For this review, take the finished solid that the model builds, in its own axes (mm). A direction names the side the tool comes from. Give positions to 0.01 mm unless a question says otherwise; leave off trailing zeros. Write each loop counter-clockwise with the first axis right and the second up, starting at its lowest first coordinate (ties: lowest second). Pieces come first, ordered by that corner, then holes.
Q1. Insertion check: P1, Ø10, axis at x = -33, z = 9.5, coming from the -Y side; P2, Ø10, axis at y = 2.5, z = 15, coming from the -X side; P3, Ø1, axis at x = -34, z = 9.5, coming from the +Y side; P4, Ø11.5, axis at x = -44.45, y = 0, coming from the -Z side. Each pin has a flat end and moves straight along its axis. Give the tip position at first contact, or say it passes through.
Q2. We need section C-C (z = 8). Write out the cut boundary in (x, y), then the cut area to 3 significant figures.
Q3. We need section D-D (x = 4.5). Write out the cut boundary in (y, z).
Q4. Machinability: for faces 1 (the flat face through (35, -19.05, 6)), 2 (the flat face through (0, -14.288, 34)), 3 (the flat face through (-35, 19.05, 6)), 4 (the flat face through (-37, 0, 12.7)), which of the approach directions +Z, -Z, +X, -X, +Y, -Y give a long, thin tool a straight path to every point of the face, cutting with its end or side? Answer none if there is none.
Q5. For line 1 (Y direction, x = -44.45, z = 7.75); line 2 (Z direction, x = -50, y = 8.5); line 3 (Y direction, x = 50.5, z = 9), list the stretches that pass through material, from the lowest coordinate up.
Q6. We need section A-A (y = 0). Write out the cut boundary in (x, z).
Q7. Mouldability with a two-part tool opening along Y and no side actions: class faces 5 (the flat face through (35, 19.05, 6)), 6 (the flat face through (-35, -19.05, 6)), 7 (the flat face through (0, 0, 25.4)), 8 (the cylindrical face through (-37.636, 2.146, 6.439)) as released by +Y, released by -Y, zero draft, split by the parting line, or undercut.
Q8. We need section B-B (x = 50). Write out the cut boundary in (y, z).
```python
from build123d import *

# Parameters (mm, degrees)
F1_DEPTH = 31.75
F2_DEPTH = 19.05
F5_DEPTH = 12.7
F6_DEPTH = 25.4
F7_DEPTH = 25.4
F8_W     = 40.1893556118
F8_H     = 22.225
F8_W_2   = 32.2620980442
F9_DEPTH = 14.2875


with BuildPart() as f1:
    # F0 (on Front) → F1 (new body, symmetric)
    with BuildSketch(Plane.XZ):
        Polygon((0, 47.625), (0, 12.7), (20.1639581514, 12.7), align=None)
        Polygon((-27.4963065702, 0), (0, 0), (0, 12.7), (-20.1639581514, 12.7), align=None)
        Polygon((0, 12.7), (0, 0), (27.4963065702, 0), (20.1639581514, 12.7), align=None)
        Polygon((-20.1639581514, 12.7), (0, 12.7), (0, 47.625), align=None)
    extrude(amount=F1_DEPTH, both=True)

    # F0 (on Front) → F2 (join, symmetric)
    with BuildSketch(Plane.XZ):
        Polygon((-27.4963065702, 0), (0, 0), (0, 12.7), (-20.1639581514, 12.7), align=None)
        Polygon((0, 12.7), (0, 0), (27.4963065702, 0), (20.1639581514, 12.7), align=None)
        Polygon((-20.1639581514, 12.7), (0, 12.7), (0, 47.625), align=None)
        Polygon((0, 47.625), (0, 12.7), (20.1639581514, 12.7), align=None)
        Polygon((-44.45, 0), (-27.4963065702, 0), (-20.1639581514, 12.7), (-44.45, 12.7), align=None)
        Polygon((20.1639581514, 12.7), (27.4963065702, 0), (44.45, 0), (44.45, 12.7), align=None)
    extrude(amount=F2_DEPTH, both=True)

    # F4 (on face) + F3 (on face) → F5 (join, through all)
    with BuildSketch(Plane.XY.offset(12.7)):
        with BuildLine():
            ThreePointArc((44.45, -19.05), (57.9203841816, -13.4703841816), (63.5, 0))
            ThreePointArc((63.5, 0), (57.9203841816, 13.4703841816), (44.45, 19.05))
            Line((44.45, 19.05), (44.45, 7.14375))
            ThreePointArc((44.45, 7.14375), (49.5013940681, 5.0513940681), (51.59375, 0))
            ThreePointArc((51.59375, 0), (49.5013940681, -5.0513940681), (44.45, -7.14375))
            Line((44.45, -7.14375), (44.45, -19.05))
        make_face()
        with BuildLine():
            Line((44.45, 7.14375), (44.45, 19.05))
            ThreePointArc((44.45, 19.05), (25.4, 0), (44.45, -19.05))
            Line((44.45, -19.05), (44.45, -7.14375))
            ThreePointArc((44.45, -7.14375), (37.30625, 0), (44.45, 7.14375))
        make_face()
    with BuildSketch(Plane.XY.offset(12.7)):
        with BuildLine():
            ThreePointArc((-44.45, -19.05), (-30.9796158184, -13.4703841816), (-25.4, 0))
            ThreePointArc((-25.4, 0), (-30.9796158184, 13.4703841816), (-44.45, 19.05))
            Line((-44.45, 19.05), (-44.45, 7.14375))
            ThreePointArc((-44.45, 7.14375), (-39.3986059319, 5.0513940681), (-37.30625, 0))
            ThreePointArc((-37.30625, 0), (-39.3986059319, -5.0513940681), (-44.45, -7.14375))
            Line((-44.45, -7.14375), (-44.45, -19.05))
        make_face()
        with BuildLine():
            Line((-44.45, 7.14375), (-44.45, 19.05))
            ThreePointArc((-44.45, 19.05), (-63.5, 0), (-44.45, -19.05))
            Line((-44.45, -19.05), (-44.45, -7.14375))
            ThreePointArc((-44.45, -7.14375), (-51.59375, 0), (-44.45, 7.14375))
        make_face()
    extrude(amount=-F5_DEPTH)

    # F3 (on face) → F6 (cut)
    with BuildSketch(Plane.XY.offset(12.7)):
        with BuildLine():
            ThreePointArc((-37.30625, 0), (-39.3986059319, 5.0513940681), (-44.45, 7.14375))
            Line((-44.45, 7.14375), (-44.45, -7.14375))
            ThreePointArc((-44.45, -7.14375), (-39.3986059319, -5.0513940681), (-37.30625, 0))
        make_face()
        with BuildLine():
            Line((-44.45, -7.14375), (-44.45, 7.14375))
            ThreePointArc((-44.45, 7.14375), (-51.59375, 0), (-44.45, -7.14375))
        make_face()
    extrude(amount=-F6_DEPTH, mode=Mode.SUBTRACT)

    # F4 (on face) → F7 (cut)
    with BuildSketch(Plane.XY.offset(12.7)):
        with BuildLine():
            Line((44.45, -7.14375), (44.45, 7.14375))
            ThreePointArc((44.45, 7.14375), (37.30625, 0), (44.45, -7.14375))
        make_face()
    extrude(amount=-F7_DEPTH, mode=Mode.SUBTRACT)

    # F8 (on Front) → F9 (cut, symmetric)
    with BuildSketch(Plane.XZ):
        with Locations((-20.0946778059, 36.5125)):
            Rectangle(F8_W, F8_H)
        with Locations((16.1310490221, 36.5125)):
            Rectangle(F8_W_2, F8_H)
    extrude(amount=F9_DEPTH, both=True, mode=Mode.SUBTRACT)


solid = f1.part
```
Computed:
1. P1: stops at y = -19.05
1. P2: stops at x = -63.5
1. P3: stops at y = 19.05
1. P4: passes through
2. outline: (-44.45, -19.05) - (-22.88, -19.05) - (-22.88, -31.75) - (22.88, -31.75) - (22.88, -19.05) - (44.45, -19.05) arc R19.05 ccw to (44.45, 19.05) - (22.88, 19.05) - (22.88, 31.75) - (-22.88, 31.75) - (-22.88, 19.05) - (-44.45, 19.05) arc R19.05 ccw to start; hole circle Ø14.29 at (-44.45, 0); hole circle Ø14.29 at (44.45, 0)
2. area: 5,370 mm2
3. outline: (-31.75, 0) - (31.75, 0) - (31.75, 39.83) - (14.29, 39.83) - (14.29, 25.4) - (-14.29, 25.4) - (-14.29, 39.83) - (-31.75, 39.83) - close
4. face 1: +Z, +X, -Y
4. face 2: +Z, +X, -X
4. face 3: +Z, -X, +Y
4. face 4: +Z, -X, +Y, -Y
5. line 1: y = -19.05 to -7.14, 7.14 to 19.05
5. line 2: z = 0 to 12.7
5. line 3: y = -18.06 to -3.8, 3.8 to 18.06
6. outline: (-63.5, 0) - (-51.59, 0) - (-51.59, 12.7) - (-63.5, 12.7) - close; (-37.31, 0) - (37.31, 0) - (37.31, 12.7) - (20.16, 12.7) - (12.83, 25.4) - (-12.83, 25.4) - (-20.16, 12.7) - (-37.31, 12.7) - close; (51.59, 0) - (63.5, 0) - (63.5, 12.7) - (51.59, 12.7) - close
7. face 5: released by +Y
7. face 6: released by -Y
7. face 7: undercut
7. face 8: undercut
8. outline: (-18.22, 0) - (-4.5, 0) - (-4.5, 12.7) - (-18.22, 12.7) - close; (4.5, 0) - (18.22, 0) - (18.22, 12.7) - (4.5, 12.7) - close
